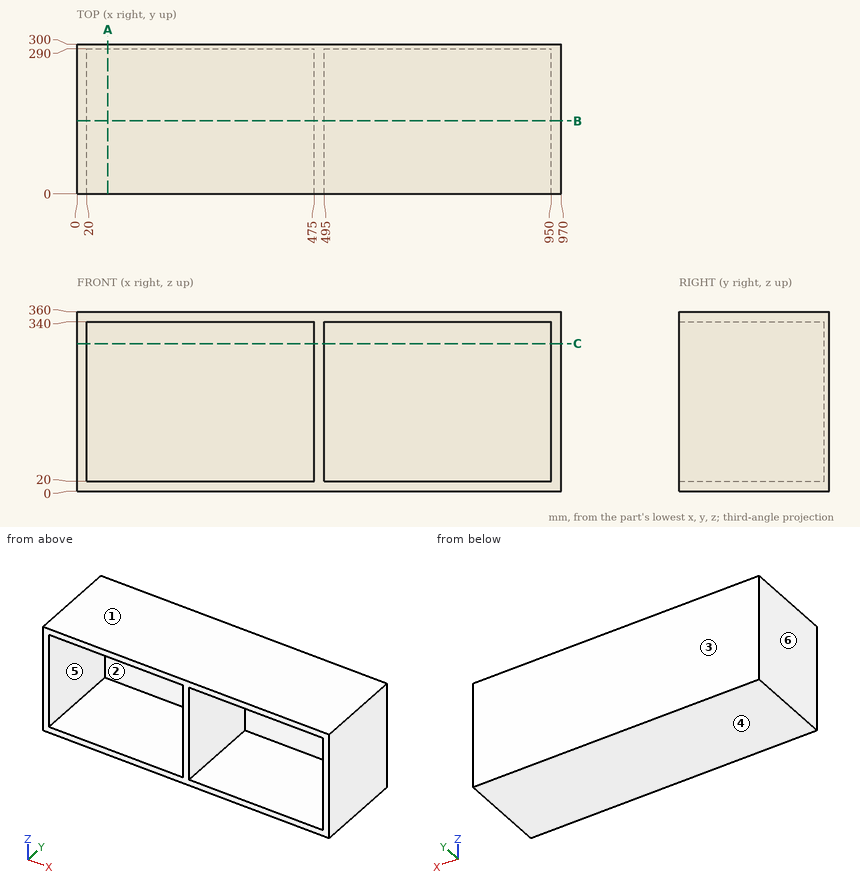
Source: three-view drawing plus pictorial views. Frame: mm from the lowest corner of the part. A direction names the side the tool comes from. Round coordinates to 2 decimals unless told otherwise and drop trailing zeros. Order: outer loops, then holes, each group sorted by start corner. A loop starts at its lowest first (then second) coordinate and runs counter-clockwise, first axis right, second up. Notation, with made-up numbers: M -28,15.25 L 31,15.25 A27 cw 31,32.25 Z; hole C 36,-12 d2. An arc over 180 degrees is marked long. One line per item, written item: value.
(1) Cut plane C-C (z = 296). Return the cut outline in (x, y), and give its area (3 significant figures).
Result sheet:
outline: M 0,0 L 20,0 L 20,290 L 475,290 L 475,0 L 495,0 L 495,290 L 950,290 L 950,0 L 970,0 L 970,300 L 0,300 Z
area: 27,100 mm2
(2) Pull-direction query (Z, two-part tool) for the marked faces 1, 2, 3 and 4; classes: pulls with the +Z half, pulls with the -Z half, needs draft (parallel to the pull), parting line crosses it, or undercut.
Result sheet:
face 1: pulls with the +Z half
face 2: undercut
face 3: needs draft
face 4: pulls with the -Z half
(3) Line query: probe 1 along X at (y, z) = (246, 170); probe 2 along Z at (x, y) = (443, 58); probe 3 along Y at (x, z) = (58, 248.5). Output: solid intervals per line, ascending. Write a range as [from, to].
Result sheet:
probe 1: [0, 20], [475, 495], [950, 970]
probe 2: [0, 20], [340, 360]
probe 3: [290, 300]
(4) Cut plane B-B (y = 146). Return the cut outline in (x, z), and give its area (3 significant figures).
Result sheet:
outline: M 0,0 L 970,0 L 970,360 L 0,360 Z; hole M 20,20 L 475,20 L 475,340 L 20,340 Z; hole M 495,20 L 950,20 L 950,340 L 495,340 Z
area: 58,000 mm2
(5) Reachability of the marked faces 5 and 6 from +Z, -Z, +X, -X, +Y, -Y: full face, straight path, thin tool, end or side. Return the list, or none.
Result sheet:
face 5: -Y
face 6: +Z, -Z, -X, +Y, -Y
(6) Pin query (flat end, axial travel): P1, Ø3, axis at x = 727, y = 73.5, coming from the -Z side; P2, Ø10, axis at x = 604, z = 150, coming from the -Y side. Return the tip coordinate at first contact, or that it passes through.
Result sheet:
P1: z = 0
P2: y = 290
(7) Cut plane A-A (x = 62). Return the cut outline in (y, z), and give its area (3 significant figures).
Result sheet:
outline: M 0,0 L 300,0 L 300,360 L 0,360 L 0,340 L 290,340 L 290,20 L 0,20 Z
area: 15,200 mm2
